```python
from build123d import *

# Parameters (mm, degrees)
SKETCH1_W             = 80
SKETCH1_H             = 110
BOSS_EXTRUDE1_DEPTH   = 20
SKETCH1_H_2           = 28
BOSS_EXTRUDE1_2_DEPTH = 20
SKETCH1_3_W           = 80
SKETCH1_3_H           = 10
SKETCH1_3_H_2         = 12
BOSS_EXTRUDE2_DEPTH   = 56
SKETCH1_4_W           = 80
SKETCH1_4_H           = 10
BOSS_EXTRUDE3_DEPTH   = 68
SKETCH2_R             = 4
BOSS_EXTRUDE4_DEPTH   = 150
SKETCH3_W             = 6
SKETCH3_H             = 170
CUT_EXTRUDE1_DEPTH    = 5


with BuildPart() as part:
    # Sketch1 → Boss-Extrude1 (new body)
    with BuildSketch(Plane(origin=(0, 0, 0), x_dir=(1, 0, 0), z_dir=(0, 1, 0))):
        with Locations((0, -20)):
            Rectangle(SKETCH1_W, SKETCH1_H)
    extrude(amount=BOSS_EXTRUDE1_DEPTH)



with BuildPart() as body_2:
    # Sketch1 → Boss-Extrude1 2 (new body)
    with BuildSketch(Plane(origin=(0, 0, 0), x_dir=(1, 0, 0), z_dir=(0, 1, 0))):
        with Locations((0, 61)):
            Rectangle(SKETCH1_W, SKETCH1_H_2)
    extrude(amount=BOSS_EXTRUDE1_2_DEPTH)


with BuildPart() as part_1:
    add(part.part)

    add(body_2.part)  # Boss-Extrude2 merges body 2
    # Sketch1_3 → Boss-Extrude2 (add)
    with BuildSketch(Plane(origin=(0, 0, 0), x_dir=(1, 0, 0), z_dir=(0, 1, 0))):
        with Locations((0, -80)):
            Rectangle(SKETCH1_3_W, SKETCH1_3_H)
        with Locations((0, 41)):
            Rectangle(SKETCH1_3_W, SKETCH1_3_H_2)
    extrude(amount=BOSS_EXTRUDE2_DEPTH)

    # Sketch1_4 → Boss-Extrude3 (add)
    with BuildSketch(Plane(origin=(0, 0, 0), x_dir=(1, 0, 0), z_dir=(0, 1, 0))):
        with Locations((0, 80)):
            Rectangle(SKETCH1_4_W, SKETCH1_4_H)
    extrude(amount=BOSS_EXTRUDE3_DEPTH)

    # Sketch2 → Boss-Extrude4 (add)
    with BuildSketch(Plane(origin=(0, 0, 75), x_dir=(-1, 0, 0), z_dir=(0, 0, -1))):
        with Locations((-30, 38)):
            Circle(SKETCH2_R)
        with Locations((30, 38)):
            Circle(SKETCH2_R)
    extrude(amount=BOSS_EXTRUDE4_DEPTH)

    # Sketch3 → Cut-Extrude1 (cut)
    with BuildSketch(Plane.XZ):
        with Locations((-30, 0)):
            Rectangle(SKETCH3_W, SKETCH3_H)
        with Locations((30, 0)):
            Rectangle(SKETCH3_W, SKETCH3_H)
    extrude(amount=-CUT_EXTRUDE1_DEPTH, mode=Mode.SUBTRACT)


solid = part_1.part
```
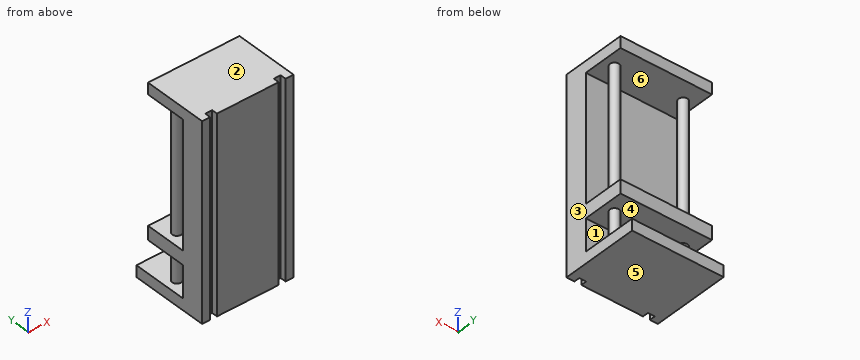
For this review, take the finished solid that the model builds, in its own axes (mm). Face numbers are marked on the shaded views. A direction names the side the tool comes from. Round coordinates to 2 decimals unless told otherwise and drop trailing zeros. Write each loop counter-clockwise with the first axis right and the second up, starting at its lowest first coordinate (ties: lowest second). Pieces come first, ordered by that corner, then holes.
1) For line 1 along Z through (x, y) = (-32, 45.5); line 2 along X through (y, z) = (4.5, -60); line 3 along Y through (x, z) = (5, 29), list the stretches that pass through material, from the lowest coordinate up.
Answer below:
line 1: z = -85 to -75, -47 to -35, 75 to 85
line 2: x = -40 to -33, -27 to 27, 33 to 40
line 3: y = 0 to 20
2) Insertion check: pin 1 Ø14 at (x, z) = (10.5, -54.5) entering from +Y; pin 2 Ø5 at (y, z) = (42.5, -51) entering from -X; pin 3 Ø5 at (x, z) = (7, 81) entering from +Y. Each pin has a flat end and moves straight along its axis. Give the tip position at first contact, or say it passes through.
Answer below:
pin 1: stops at y = 20
pin 2: stops at x = -33.46
pin 3: stops at y = 56
3) Take a section at C-C on y = 38. Give the boundary of the cut face in (x, z), then the cut area to 3 significant figures.
Answer below:
outline: (-40, -85) - (40, -85) - (40, -75) - (34, -75) - (34, -47) - (40, -47) - (40, -35) - (34, -35) - (34, 75) - (40, 75) - (40, 85) - (-40, 85) - (-40, 75) - (-34, 75) - (-34, -35) - (-40, -35) - (-40, -47) - (-34, -47) - (-34, -75) - (-40, -75) - close; hole (-26, -75) - (26, -75) - (26, -47) - (-26, -47) - close; hole (-26, -35) - (26, -35) - (26, 75) - (-26, 75) - close
area: 4,770 mm2
4) Take a section at B-B on z = -15. Give the boundary of the cut face in (x, y), then the cut area to 3 significant figures.
Answer below:
outline: (-40, 0) - (-33, 0) - (-33, 5) - (-27, 5) - (-27, 0) - (27, 0) - (27, 5) - (33, 5) - (33, 0) - (40, 0) - (40, 20) - (-40, 20) - close; circle Ø8 at (-30, 38); circle Ø8 at (30, 38)
area: 1,640 mm2
5) Mouldability with a two-part tool opening along Z and no side actions: class the marked faces 3, 4, 5 and 6 as +Z half, -Z half, draft (parallel to the pull), parting line (faces both ways), or undercut.
Answer below:
face 3: draft
face 4: undercut
face 5: -Z half
face 6: undercut
6) Machinability: for the marked faces 1 and 2, which of the approach directions +Z, -Z, +X, -X, +Y, -Y give a long, thin tool a straight path to every point of the face, cutting with its end or side? Answer none if there is none.
Answer below:
face 1: +X, -X
face 2: +Z, +X, -X, +Y, -Y
7) Take a section at D-D on x = 30. Give the boundary of the cut face in (y, z).
Answer below:
outline: (5, -85) - (68, -85) - (68, -75) - (42, -75) - (42, -47) - (56, -47) - (56, -35) - (42, -35) - (42, 75) - (56, 75) - (56, 85) - (5, 85) - close; hole (20, -75) - (34, -75) - (34, -47) - (20, -47) - close; hole (20, -35) - (34, -35) - (34, 75) - (20, 75) - close
8) Take a section at A-A on y = 49. Give the boundary of the cut face in (x, z).
Answer below:
outline: (-40, -85) - (40, -85) - (40, -75) - (-40, -75) - close; (-40, -47) - (40, -47) - (40, -35) - (-40, -35) - close; (-40, 75) - (40, 75) - (40, 85) - (-40, 85) - close
